Verification items for the finished model (mm, model axes). Face numbers are marked on the shaded views. Coordinates: 2 decimals unless noted, no trailing zeros. Write each loop counter-clockwise with the first axis right and the second up, starting at its lowest first coordinate (ties: lowest second). Pieces come first, ordered by that corner, then holes. Notation, with made-up numbers: (30, 38.5) -> (43, 38.5) arc R15 ccw to (43, 51.5) -> close; hole circle Ø9 at (59, -9.5). An arc over 180 degrees is marked (long way). Write each question's results on one line, items separated by ' | '. Start each with the question number.
from build123d import *

# Parameters (mm, degrees)
F1_DEPTH = 12.7
F2_R     = 3.81
F3_DEPTH = 15.876
F4_SIZE  = 2.54


with BuildPart() as f1:
    # F0 (on Top) → F1 (new body, symmetric)
    with BuildSketch(Plane.XY):
        Polygon((-23.495, 15.875), (-7.62, 0), (7.62, 0), (23.495, 15.875), align=None)
    extrude(amount=F1_DEPTH, both=True)

    # F2 (on Front) → F3 (cut, through all)
    with BuildSketch(Plane.XZ):
        Circle(F2_R)
    extrude(amount=-F3_DEPTH, mode=Mode.SUBTRACT)

    # F4
    f4_edges = [f1.edges().sort_by_distance(p)[0] for p in [
        (-23.495, 15.875, 0),
        (23.495, 15.875, 0),
    ]]
    chamfer(f4_edges, length=F4_SIZE)


solid = f1.part
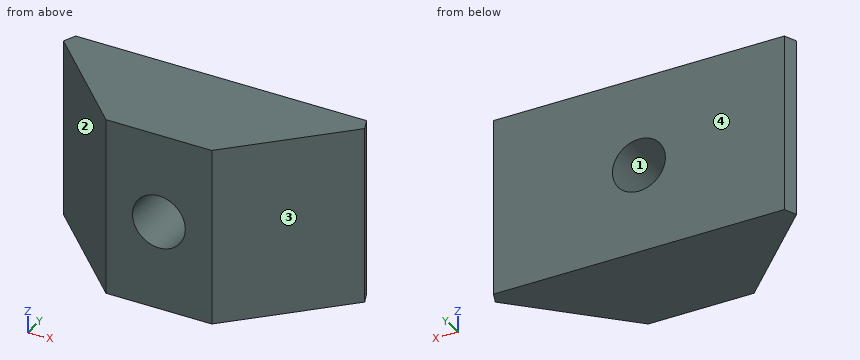
1. Material ranges on probe 1 along Z at (x, y) = (0, 3.5); probe 2 along X at (y, z) = (7, 2.25); probe 3 along Y at (x, z) = (-9.5, -5) (3 decimals), recorded low to high. Write a range as from..to.
2. Sectioned sample at A-A on x = 0. Record the cut outline in (y, z) (3 decimals).
3. Mould release check, pull along X, two halves, no side actions. Record for the marked faces 1, 2, 3 and 4: +X half, -X half, draft (parallel to the pull), parting line (faces both ways), or undercut.
4. Depth check by flat-ended pin: pin 1 Ø3 at (y, z) = (12, 0) entering from +X; pin 2 Ø3 at (y, z) = (8.5, 6.5) entering from +X; pin 3 Ø8 at (y, z) = (4.5, -2) entering from +X. Enter the tip coordinate at first touch or a pass-through.
5. Sectioned sample at C-C on y = 3.75. Record the cut outline in (x, z).
6. Sectioned sample at D-D on z = -10.5. Record the cut outline in (x, y) (3 decimals), plus the area to 3 significant figures.
7. Sectioned sample at B-B on z = 0. Record the cut outline in (x, y) (3 decimals), plus the area to 3 significant figures.
Computed values:
1) probe 1: z = -12.7..-3.81, 3.81..12.7 | probe 2: x = -14.62..-3.07, 3.07..14.62 | probe 3: y = 1.88..15.875
2) outline: (0, -12.7) -> (15.875, -12.7) -> (15.875, -3.81) -> (0, -3.81) -> close; (0, 3.81) -> (15.875, 3.81) -> (15.875, 12.7) -> (0, 12.7) -> close
3) face 1: undercut | face 2: -X half | face 3: +X half | face 4: draft
4) pin 1: stops at x = 21.12 | pin 2: stops at x = 17.62 | pin 3: stops at x = 16.12
5) outline: (-11.37, -12.7) -> (11.37, -12.7) -> (11.37, 12.7) -> (-11.37, 12.7) -> close; hole circle Ø7.62 at (0, 0)
6) outline: (-21.699, 14.079) -> (-7.62, 0) -> (7.62, 0) -> (21.699, 14.079) -> (20.955, 15.875) -> (-20.955, 15.875) -> close | area: 489 mm^2
7) outline: (-21.699, 14.079) -> (-7.62, 0) -> (-3.81, 0) -> (-3.81, 15.875) -> (-20.955, 15.875) -> close; (3.81, 0) -> (7.62, 0) -> (21.699, 14.079) -> (20.955, 15.875) -> (3.81, 15.875) -> close | area: 368 mm^2
